Geometry: final body of the model. Coordinates: model frame, mm. A direction names the side the tool comes from. Round coordinates to 2 decimals unless told otherwise and drop trailing zeros. Order: outer loops, then holes, each group sorted by start corner. A loop starts at its lowest first (then second) coordinate and runs counter-clockwise, first axis right, second up. Notation, with made-up numbers: (-3, 67.5) - (55, 67.5) arc R14 cw to (55, 75.5) - close; hole circle Ø8 at (39.25, 22). An arc over 180 degrees is marked (long way). Put each result on its own line as item: value. Start each with the question number.
(1) Pin query (flat end, axial travel): P1, Ø1, axis at y = 7, z = 1.5, coming from the +X side; P2, Ø2, axis at x = 0.5, z = 1, coming from the +Y side; P3, Ø1, axis at x = 1.5, z = 0.5, coming from the -Y side. Return the tip coordinate at first contact, or that it passes through.
(2) Section C-C (z = 1.5). Output: boundary loops of the cut face in (x, y), and give its area (3 significant figures).
(3) Access query for faces 1 (the face through (-1.5, 7.5, 3)), 2 (the face through (0, 0, 4)). Directions: +Z, -Z, +X, -X, +Y, -Y. A direction counts if a zero-diameter tool reaches every point of the face in a straight line with its end or side. Return the directions, or none.
(4) Material intervals for L1, parallel to Z at x = 1.5, y = 8; L2, parallel to X at y = -0.5, z = 1.6; L3, parallel to Y at x = -3, z = 3.2, sorted ascending. Write a range as [from, to].
(5) Section A-A (x = 0). Output: boundary loops of the cut face in (y, z), and give its area (3 significant figures).
from build123d import *

# Parameters (mm, degrees)
F0_R     = 7.45
F1_DEPTH = 3
F2_R     = 10
F2_R_2   = 7.45
F3_DEPTH = 1
F4_SIZE  = 0.75
F5_SIZE  = 0.5


with BuildPart() as f1:
    # F0 (on Top) → F1 (new body)
    with BuildSketch(Plane.XY):
        Circle(F0_R)
    extrude(amount=F1_DEPTH)

    # F2 (on face) → F3 (join)
    with BuildSketch(Plane.XY.offset(3)):
        Circle(F2_R)
        Circle(F2_R_2, mode=Mode.SUBTRACT)
        Circle(F2_R_2)
    extrude(amount=F3_DEPTH)

    # F4
    f4_edges = [f1.edges().sort_by_distance(p)[0] for p in [
        (-7.45, 0, 0),
    ]]
    chamfer(f4_edges, length=F4_SIZE)

    # F5
    f5_edges = [f1.edges().sort_by_distance(p)[0] for p in [
        (-10, 0, 4),
    ]]
    chamfer(f5_edges, length=F5_SIZE)


solid = f1.part
Checks:
1. P1: stops at x = 3.64
1. P2: stops at y = 7.45
1. P3: stops at y = -7.37
2. outline: circle Ø14.9 at (0, 0)
2. area: 174 mm²
3. face 1: -Z
3. face 2: +Z, +X, -X, +Y, -Y
4. L1: z = [3, 4]
4. L2: x = [-7.43, 7.43]
4. L3: y = [-9.54, 9.54]
5. outline: (-10, 3) - (-7.45, 3) - (-7.45, 0.75) - (-6.7, 0) - (6.7, 0) - (7.45, 0.75) - (7.45, 3) - (10, 3) - (10, 3.5) - (9.5, 4) - (-9.5, 4) - (-10, 3.5) - close
5. area: 63.9 mm²
